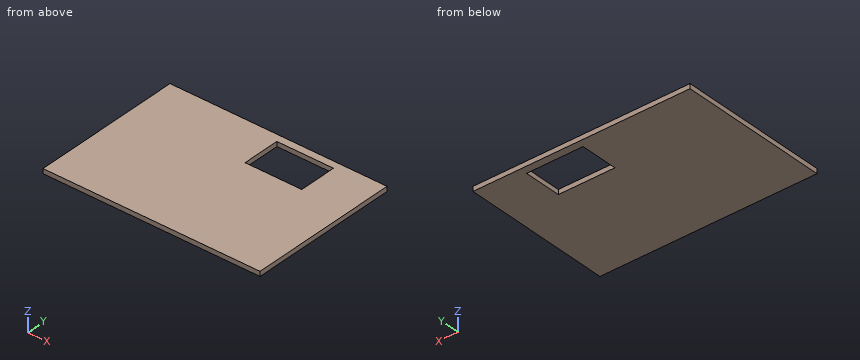
```python
from build123d import *

# Parameters (mm, degrees)
BOX013_W     = 30
BOX013_H     = 20
BOX013_DEPTH = 2.5
BOX012_W     = 115
BOX012_H     = 80
BOX012_DEPTH = 2.5


with BuildPart() as cubo005:
    # Box013 → Box013 (new body)
    with BuildSketch(Plane(origin=(60, 56, 25), x_dir=(1, 0, 0), z_dir=(0, 0, 1))):
        with Locations((15, 10)):
            Rectangle(BOX013_W, BOX013_H)
    extrude(amount=BOX013_DEPTH)


with BuildPart() as cut017:
    # Box012 → Box012 (new body)
    with BuildSketch(Plane.XY.offset(25)):
        with Locations((57.5, 40)):
            Rectangle(BOX012_W, BOX012_H)
    extrude(amount=BOX012_DEPTH)

    # Cut017: cut Cubo005
    add(cubo005.part, mode=Mode.SUBTRACT)


solid = cut017.part
```
The listing builds one solid part. Answer for the finished solid, in the listing's coordinates (mm). Give positions to 0.01 mm unless a question says otherwise; leave off trailing zeros. Write each loop counter-clockwise with the first axis right and the second up, starting at its lowest first coordinate (ties: lowest second). Pieces come first, ordered by that corner, then holes. Notation, with made-up numbers: (66.25, -27) - (84.25, -27) arc R28 cw to (84.25, 6) - close; hole circle Ø8 at (-3, 27). An arc over 180 degrees is marked (long way). Use one line per item in the form item = value. Start each with the question number.
1) Find section C-C on z = 26.55. Determine the outline of the cut face in (x, y).
2) Find section B-B on x = 82. Determine the outline of the cut face in (y, z).
3) Find section A-A on y = 59. Determine the outline of the cut face in (x, z), plus the area to 4 significant figures.
4) Consider line 1 along Y through (x, z) = (63.5, 26.3); line 2 along X through (y, z) = (62.5, 25.35). Determine where each line is inside the solid, lowest interval first. Write a range as from..to.
Geometry results:
q1.outline = (0, 0) - (115, 0) - (115, 80) - (0, 80) - close; hole (60, 56) - (90, 56) - (90, 76) - (60, 76) - close
q2.outline = (0, 25) - (56, 25) - (56, 27.5) - (0, 27.5) - close; (76, 25) - (80, 25) - (80, 27.5) - (76, 27.5) - close
q3.outline = (0, 25) - (60, 25) - (60, 27.5) - (0, 27.5) - close; (90, 25) - (115, 25) - (115, 27.5) - (90, 27.5) - close
q3.area = 212.5 mm2
q4.line_1 = 0..56, 76..80
q4.line_2 = 0..60, 90..115
